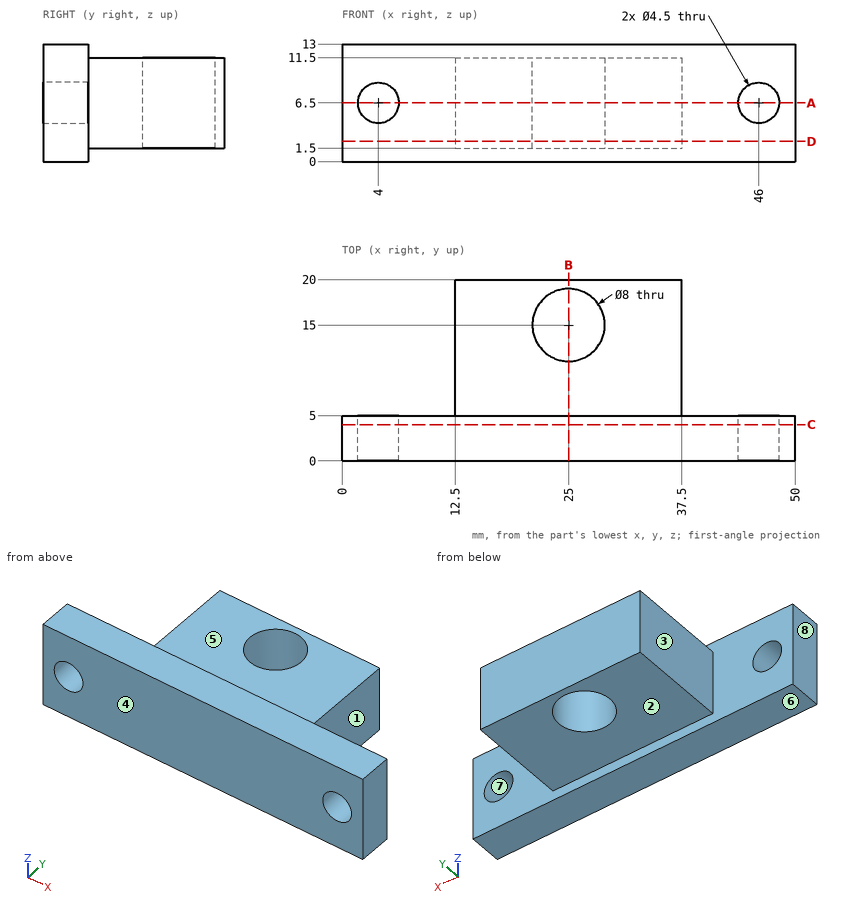
Verification items for this drawing (mm, ordinates from the low corner). A direction names the side the tool comes from. Coordinates: 2 decimals unless noted, no trailing zeros. Write each loop counter-clockwise with the first axis right and the second up, starting at its lowest first coordinate (ties: lowest second). Pieces come first, ordered by that corner, then holes. Notation, with made-up numbers: M -26.75,78 L -9.75,78 A18 cw -9.75,88 Z; hole C 69,26.5 d8. An arc over 180 degrees is marked long. Use CSV: the item, a comma, the result in double quotes.
Q1. Thickness scan on line 1 along X through (y, z) = (3.7, 6.5); line 2 along X through (y, z) = (1.5, 5.5); line 3 along X through (y, z) = (10.25, 6). Record the ranges inside material, lowest first. Write a range as [from, to].
Computed values:
line 1,"[0, 1.75], [6.25, 43.75], [48.25, 50]"
line 2,"[0, 1.98], [6.02, 43.98], [48.02, 50]"
line 3,"[12.5, 37.5]"
Q2. Go/stop test with flat-tipped pins: P1, Ø12, axis at x = 30, y = 9.5, coming from the -Z side; P2, Ø2.5, axis at x = 46, z = 6.5, coming from the -Y side; P3, Ø10.5, axis at x = 25, y = 15, coming from the +Z side. Record where each tip stops, or that it passes through.
Computed values:
P1,"z = 0"
P2,"through"
P3,"z = 11.5"
Q3. Mould release check, pull along Z, two halves, no side actions. Record for the marked faces 6, 7 and 8: pulls with the +Z half, pulls with the -Z half, needs draft (parallel to the pull), parting line crosses it, or undercut.
Computed values:
face 6,"pulls with the -Z half"
face 7,"undercut"
face 8,"needs draft"
Q4. Section check D-D, the plane z = 2.25. Enter the section's corners in (x, y), and give its area (3 significant figures).
Computed values:
outline,"M 0,0 L 50,0 L 50,5 L 37.5,5 L 37.5,20 L 12.5,20 L 12.5,5 L 0,5 Z; hole C 25,15 d8"
area,"575 mm²"
Q5. Section check A-A, the plane z = 6.5. Enter the section's corners in (x, y).
Computed values:
outline,"M 0,0 L 1.75,0 L 1.75,5 L 0,5 Z; M 6.25,0 L 43.75,0 L 43.75,5 L 37.5,5 L 37.5,20 L 12.5,20 L 12.5,5 L 6.25,5 Z; M 48.25,0 L 50,0 L 50,5 L 48.25,5 Z; hole C 25,15 d8"
Q6. Section check C-C, the plane y = 4. Enter the section's corners in (x, z).
Computed values:
outline,"M 0,0 L 50,0 L 50,13 L 0,13 Z; hole C 4,6.5 d4.5; hole C 46,6.5 d4.5"
Q7. Set-up check for the marked faces 1, 2, 3, 4 and 5: record each of +Z, -Z, +X, -X, +Y, -Y from which the full face is reachable in a straight line by a thin tool's end or side.
Computed values:
face 1,"+Z, -Z, +X, +Y"
face 2,"-Z, +X, -X, +Y"
face 3,"+Z, -Z, -X, +Y"
face 4,"+Z, -Z, +X, -X, -Y"
face 5,"+Z, +X, -X, +Y"
Q8. Section check B-B, the plane x = 25. Enter the section's corners in (y, z), and give its area (3 significant figures).
Computed values:
outline,"M 0,0 L 5,0 L 5,1.5 L 11,1.5 L 11,11.5 L 5,11.5 L 5,13 L 0,13 Z; M 19,1.5 L 20,1.5 L 20,11.5 L 19,11.5 Z"
area,"135 mm²"
